Part print with two shaded views. Sizes in mm from the minimum x, y, z corner. A direction names the side the tool comes from. Coordinates: 2 decimals unless noted, no trailing zeros. Loops run counter-clockwise (first coordinate to the right, second up) from the corner with the lowest first, then second, coordinate; pieces in that order, holes last.
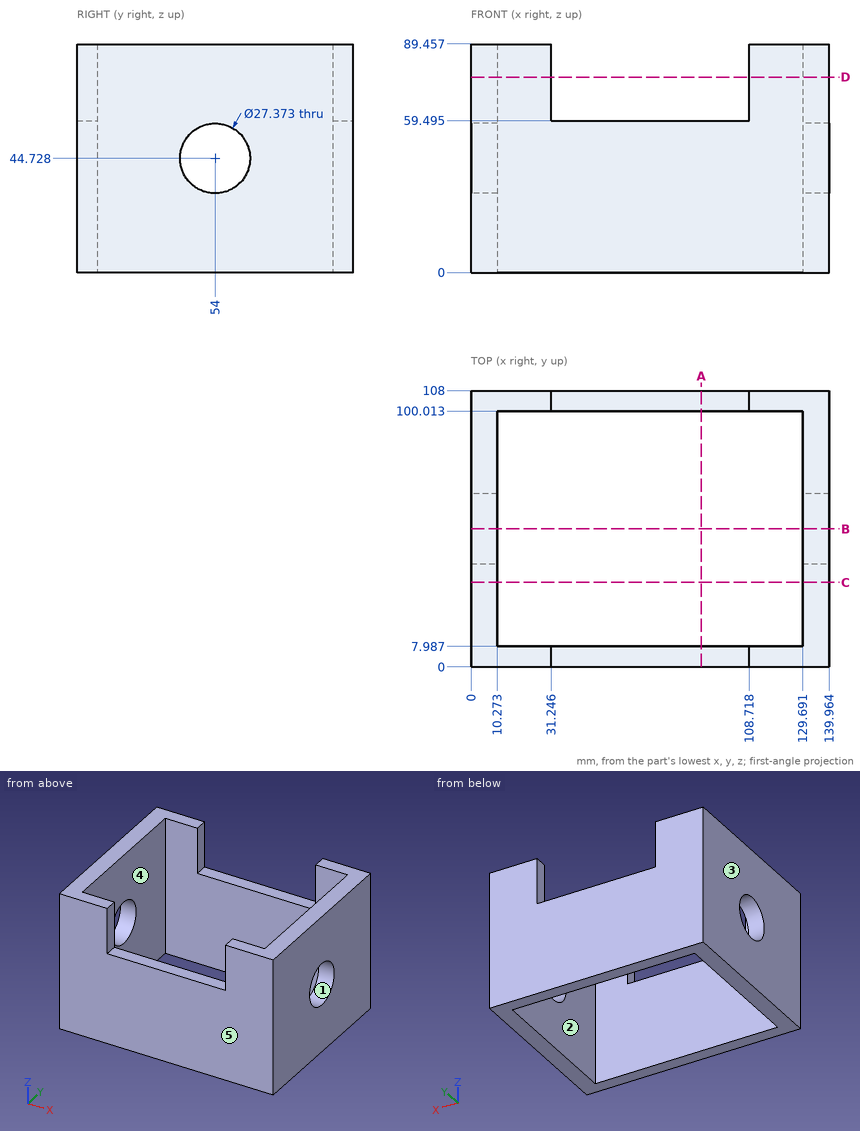
Q1. Slice it at B-B (y = 54). List the corners of the cut face in (x, z) (1 decimal), and give its area (3 significant figures).
Answers:
outline: (0, 0) - (10.3, 0) - (10.3, 31) - (0, 31) - close; (0, 58.4) - (10.3, 58.4) - (10.3, 89.5) - (0, 89.5) - close; (129.7, 0) - (140, 0) - (140, 31) - (129.7, 31) - close; (129.7, 58.4) - (140, 58.4) - (140, 89.5) - (129.7, 89.5) - close
area: 1,280 mm2
Q2. Mould opens along X. For the marked faces 1, 2 and 3 say: +X half, -X half, draft (parallel to the pull), parting line (faces both ways), or undercut.
Answers:
face 1: draft
face 2: undercut
face 3: -X half
Q3. Slice it at A-A (x = 90). List the corners of the cut face in (y, z) (1 decimal).
Answers:
outline: (0, 0) - (8, 0) - (8, 59.5) - (0, 59.5) - close; (100, 0) - (108, 0) - (108, 59.5) - (100, 59.5) - close
Q4. Which spindle directions (+Z, -Z, +X, -X, +Y, -Y) get a long thin tool onto all of the face, cutting with end or side? Do the marked faces 4 and 5. Say none if no direction does.
Answers:
face 4: +Z, -Z
face 5: +Z, -Z, +X, -X, -Y
Q5. Slice it at C-C (y = 33). List the corners of the cut face in (x, z), and give its area (3 significant figures).
Answers:
outline: (0, 0) - (10.27, 0) - (10.27, 89.46) - (0, 89.46) - close; (129.69, 0) - (139.96, 0) - (139.96, 89.46) - (129.69, 89.46) - close
area: 1,840 mm2
Q6. Flat gauge pins, fed straight in: P1, Ø3, axis at x = 105.5, z = 73.5, coming from the +Y side; P2, Ø6, axis at y = 18.5, z = 73.5, coming from the -X side; P3, Ø4, axis at x = 81, y = 4.5, coming from the +Z side (1 decimal). Where does each tip first touch, or does it go through?
Answers:
P1: passes through
P2: stops at x = 0
P3: stops at z = 59.5
Q7. Drill centre lines: line 1 (Y direction, x = 126.5, z = 39); line 2 (Z direction, x = 132, y = 54) (1 decimal); line 3 (X direction, y = 71.5, z = 54.5). Where is each one in solid material? Low to high.
Answers:
line 1: y = 0 to 7.99, 100.01 to 108
line 2: z = 0 to 31, 58.4 to 89.5
line 3: x = 0 to 10.27, 129.69 to 139.96
Q8. Slice it at D-D (z = 76.5). List the corners of the cut face in (x, y) (1 decimal), and give its area (3 significant figures).
Answers:
outline: (0, 0) - (31.2, 0) - (31.2, 8) - (10.3, 8) - (10.3, 100) - (31.2, 100) - (31.2, 108) - (0, 108) - close; (108.7, 0) - (140, 0) - (140, 108) - (108.7, 108) - (108.7, 100) - (129.7, 100) - (129.7, 8) - (108.7, 8) - close
area: 2,890 mm2
